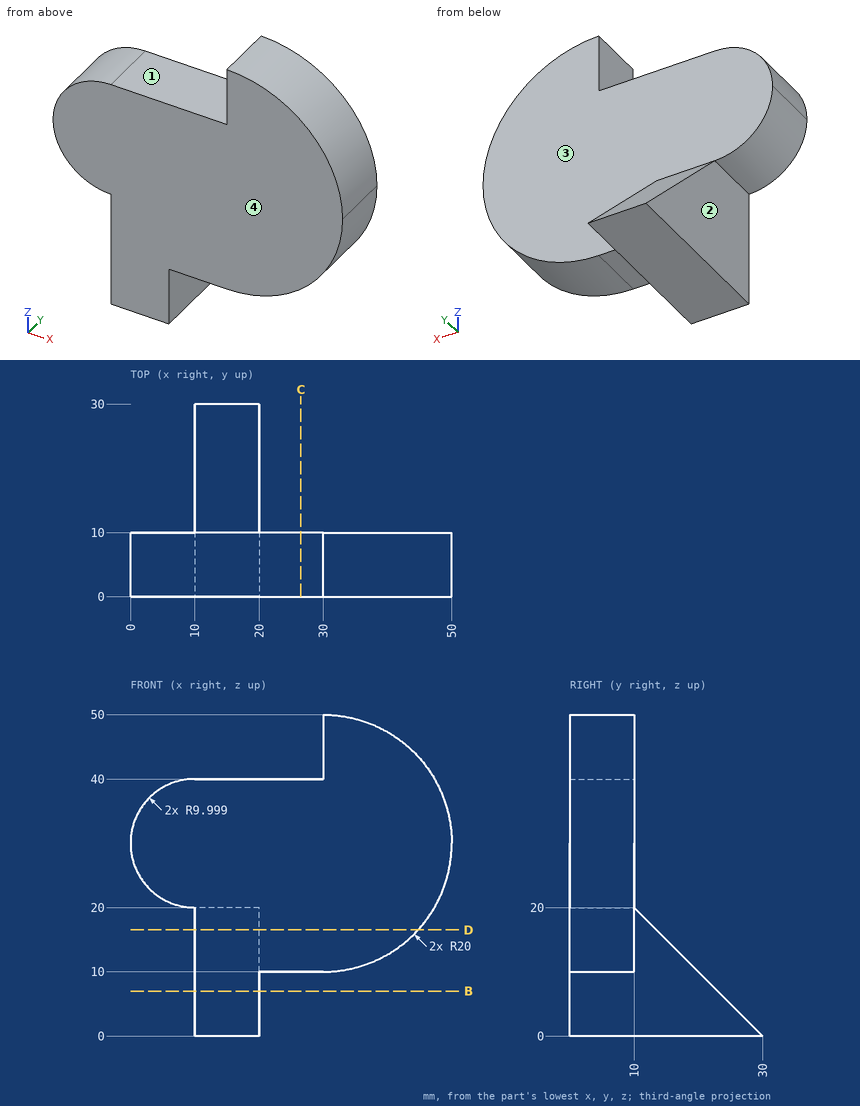
Answer from the drawing. Dimensions are ordinates in mm from the lowest x, y and z of the part. A direction names the side the tool comes from. Give positions to 0.01 mm unless a question says otherwise; leave off trailing zeros. Loops run counter-clockwise (first coordinate to the right, second up) from the corner with the lowest first, then second, coordinate; pieces in that order, holes last. Notation, with made-up numbers: (-5, 80) -> (-1, 80) arc R27 ccw to (-1, 112) -> close; hole circle Ø9 at (-6, 62). An arc over 180 degrees is marked (long way). One line per question, with ' | ' between items. Start each with the question number.
1) Section C-C, the plane x = 26.5 is taken. Determine the outline of the cut face in (y, z), then the cut area to 3 significant figures.
2) Section B-B, the plane z = 7 is taken. Determine the outline of the cut face in (x, y).
3) For the marked faces 1, 2, 3 and 4, determine the directions among +Z, -Z, +X, -X, +Y, -Y from which every point of the face is accessible in a straight line to the end or side of a thin tool.
4) Straight lines are drawn through the part: L1, parallel to Y at x = 34.5, z = 41; L2, parallel to Z at x = 20.5, y = 6; L3, parallel to Z at x = 14, y = 21.5. For each, find the intervals that lie inside material, in ascending order.
5) Section D-D, the plane z = 16.5 is taken. Determine the outline of the cut face in (x, y).
6) Each of these flat-tipped pins is pushed along its axis until it touches: pin 1 (16 mm diameter, centred on y = 12, z = 13.5, fed in from -X) (1 decimal); pin 2 (6 mm diameter, centred on y = 7.5, z = 11.5, fed in from -X); pin 3 (3 mm diameter, centred on x = 27, y = 6.5, fed in from -Z); pin 4 (10 mm diameter, centred on y = 23.5, z = 19.5, fed in from -X). Where does it stop, or does it pass through?
Resolved:
1) outline: (0, 10) -> (10, 10) -> (10, 40) -> (0, 40) -> close | area: 300 mm2
2) outline: (10, 0) -> (20, 0) -> (20, 23) -> (10, 23) -> close
3) face 1: +Z, -X, +Y, -Y | face 2: -Z, -X, +Y, -Y | face 3: +Z, +X, +Y | face 4: +Z, -Z, +X, -X, -Y
4) L1: 0 to 10 | L2: 10 to 40 | L3: 0 to 8.5
5) outline: (10, 0) -> (44.76, 0) -> (44.76, 10) -> (20, 10) -> (20, 13.5) -> (10, 13.5) -> close
6) pin 1: x = 5.2 | pin 2: x = 10 | pin 3: z = 10 | pin 4: through
